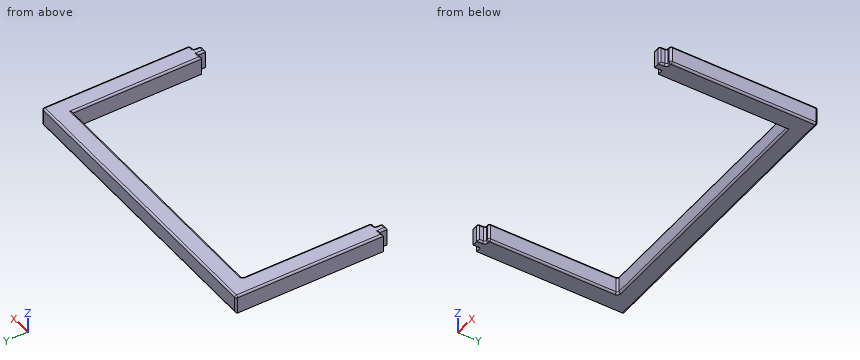
```python
from build123d import *

# Parameters (mm, degrees)
SKETCH1_W           = 2
SKETCH1_H           = 2
BOSS_EXTRUDE1_DEPTH = 5
FILLET1_R           = 0.5


with BuildPart() as part:
    # Sketch1 → Boss-Extrude1 (new body)
    with BuildSketch(Plane.XY):
        Polygon((265.633757962, -112.866242038), (185.633757962, -112.866242038), (185.633757962, -152.866242038), (187.133757962, -152.866242038), (189.133757962, -152.866242038), (190.633757962, -152.866242038), (190.633757962, -117.866242038), (260.633757962, -117.866242038), (260.633757962, -152.866242038), (262.133757962, -152.866242038), (264.133757962, -152.866242038), (265.633757962, -152.866242038), align=None)
        with Locations((188.133757962, -153.866242038)):
            Rectangle(SKETCH1_W, SKETCH1_H)
        with Locations((263.133757962, -153.866242038)):
            Rectangle(SKETCH1_W, SKETCH1_H)
    extrude(amount=BOSS_EXTRUDE1_DEPTH)

    # Fillet1
    fillet1_edges = [part.edges().sort_by_distance(p)[0] for p in [
        (262.133757962, -153.866242038, 5),
        (225.633757962, -117.866242038, 0),
        (190.633757962, -135.366242038, 0),
        (263.133757962, -154.866242038, 5),
        (189.883757962, -152.866242038, 0),
        (189.133757962, -153.866242038, 0),
        (225.633757962, -112.866242038, 0),
        (265.633757962, -132.866242038, 0),
        (264.133757962, -153.866242038, 5),
        (264.883757962, -152.866242038, 0),
        (264.133757962, -153.866242038, 0),
        (264.883757962, -152.866242038, 5),
        (265.633757962, -132.866242038, 5),
        (190.633757962, -117.866242038, 2.5),
        (190.633757962, -152.866242038, 2.5),
        (189.133757962, -152.866242038, 2.5),
        (189.133757962, -154.866242038, 2.5),
        (185.633757962, -112.866242038, 2.5),
        (265.633757962, -112.866242038, 2.5),
        (265.633757962, -152.866242038, 2.5),
        (264.133757962, -152.866242038, 2.5),
        (264.133757962, -154.866242038, 2.5),
        (225.633757962, -112.866242038, 5),
        (185.633757962, -132.866242038, 5),
        (260.633757962, -135.366242038, 5),
        (186.383757962, -152.866242038, 5),
        (187.133757962, -153.866242038, 5),
        (188.133757962, -154.866242038, 5),
        (189.133757962, -153.866242038, 5),
        (189.883757962, -152.866242038, 5),
        (190.633757962, -135.366242038, 5),
        (225.633757962, -117.866242038, 5),
        (261.383757962, -152.866242038, 5),
    ]]
    fillet(fillet1_edges, radius=FILLET1_R)


solid = part.part
```
For this review, take the finished solid that the model builds, in its own axes (mm). Give positions to 0.01 mm unless a question says otherwise; leave off trailing zeros. Order: outer loops, then holes, each group sorted by start corner. A loop starts at its lowest first (then second) coordinate and runs counter-clockwise, first axis right, second up.
1) Take a section at A-A (y = -141). Give the boundary of the cut face in (x, z), then the cut area to 3 significant figures.
2) Insertion check: pin 1 (0.8 mm diameter, centred on x = 186.5, z = 2, fed in from -Y); pin 2 (3 mm diameter, centred on x = 229.5, z = 2.5, fed in from -Y); pin 3 (1.6 mm diameter, centred on y = -154, z = 1.5, fed in from -X). Each pin has a flat end and moves straight along its axis. Give the tip position at first contact, or say it passes through.
3) Take a section at B-B (z = 3.4). Give the boundary of the cut face in (x, y).
4) Wall thickness on line 1 (X direction, y = -122, z = 2.75); line 2 (Y direction, x = 215.5, z = 4.4); line 3 (X direction, y = -116.5, z = 0.4): over which ranges is each line inside the solid? List them lowest first.
5) Take a section at C-C (x = 248). Give the boundary of the cut face in (y, z), then the cut area to 3 significant figures.
Derived:
1. outline: (185.63, 0) - (190.13, 0) arc R0.5 ccw to (190.63, 0.5) - (190.63, 4.5) arc R0.5 ccw to (190.13, 5) - (186.13, 5) arc R0.5 ccw to (185.63, 4.5) - close; (260.63, 0) - (265.13, 0) arc R0.5 ccw to (265.63, 0.5) - (265.63, 4.5) arc R0.5 ccw to (265.13, 5) - (261.13, 5) arc R0.5 ccw to (260.63, 4.5) - close
1. area: 49.7 mm2
2. pin 1: stops at y = -152.87
2. pin 2: stops at y = -117.87
2. pin 3: stops at x = 187.13
3. outline: (185.63, -152.87) - (187.13, -152.87) - (187.13, -154.87) - (188.63, -154.87) arc R0.5 ccw to (189.13, -154.37) - (189.13, -153.37) arc R0.5 cw to (189.63, -152.87) - (190.13, -152.87) arc R0.5 ccw to (190.63, -152.37) - (190.63, -118.37) arc R0.5 cw to (191.13, -117.87) - (260.63, -117.87) - (260.63, -152.87) - (262.13, -152.87) - (262.13, -154.87) - (263.63, -154.87) arc R0.5 ccw to (264.13, -154.37) - (264.13, -153.37) arc R0.5 cw to (264.63, -152.87) - (265.13, -152.87) arc R0.5 ccw to (265.63, -152.37) - (265.63, -113.37) arc R0.5 ccw to (265.13, -112.87) - (186.13, -112.87) arc R0.5 ccw to (185.63, -113.37) - close
4. line 1: x = 185.63 to 190.63, 260.63 to 265.63
4. line 2: y = -117.87 to -112.87
4. line 3: x = 185.63 to 265.62
5. outline: (-117.87, 0.5) arc R0.5 ccw to (-117.37, 0) - (-113.37, 0) arc R0.5 ccw to (-112.87, 0.5) - (-112.87, 4.5) arc R0.5 ccw to (-113.37, 5) - (-117.37, 5) arc R0.5 ccw to (-117.87, 4.5) - close
5. area: 24.8 mm2
